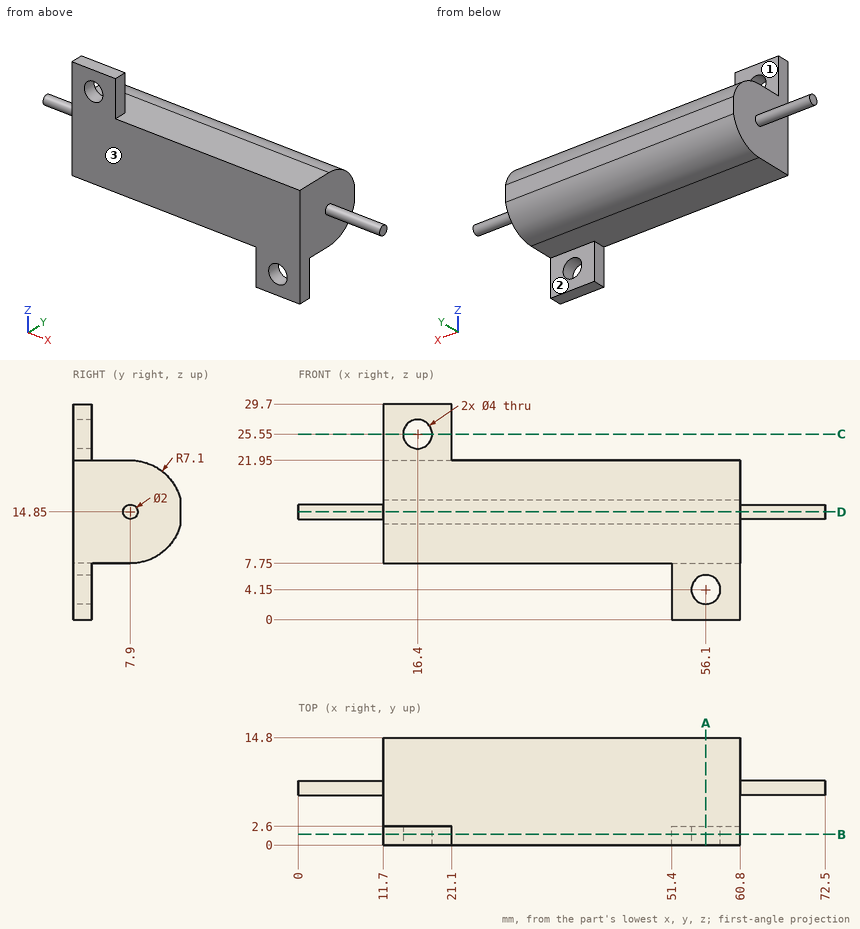
Design review of the part shown in the three views and the two pictorial views. Dimensions are in mm from the part's minimum x, y and z. A direction names the side the tool comes from. Coordinates: 2 decimals unless noted, no trailing zeros. Write each loop counter-clockwise with the first axis right and the second up, starting at its lowest first coordinate (ties: lowest second). Pieces come first, ordered by that corner, then holes. Notation, with made-up numbers: (-20, 84) - (35, 84) arc R13 ccw to (35, 99) - close; hole circle Ø5 at (-19.75, -7). An arc over 180 degrees is marked (long way). Write item = value, one per line.
(1) For P1, Ø4.5, axis at y = 5.5, z = 23, coming from the -X side; P2, Ø1.3, axis at y = 2, z = 24.5, coming from the +X side; P3, Ø3, axis at x = 54.5, y = 6, coming from the -Z side; P4, Ø3, axis at x = 56.1, z = 4.15, coming from the +Y side, all flat-tipped, find the tip position at first contact; note any pin that passes through.
Result sheet:
P1 = 11.7
P2 = 21.1
P3 = 7.75
P4 = through
(2) Consider section B-B, the plane y = 1.5. Give the boundary of the cut face in (x, z), then the cut area to 3 significant figures.
Result sheet:
outline = (11.7, 7.75) - (51.4, 7.75) - (51.4, 0) - (60.8, 0) - (60.8, 21.95) - (21.1, 21.95) - (21.1, 29.7) - (11.7, 29.7) - close; hole circle Ø4 at (16.4, 25.55); hole circle Ø4 at (56.1, 4.15)
area = 818 mm^2
(3) For line 1 (Z direction, x = 16.4, y = 1); line 2 (Z direction, x = 38, y = 1.5); line 3 (X direction, y = 3.25, z = 18.5), list the stretches that pass through material, from the lowest coordinate up. Write a range as [from, to].
Result sheet:
line_1 = [7.75, 23.55], [27.55, 29.7]
line_2 = [7.75, 21.95]
line_3 = [11.7, 60.8]
(4) Consider section D-D, the plane z = 14.85. Give the boundary of the cut face in (x, y).
Result sheet:
outline = (0, 6.9) - (11.7, 6.9) - (11.7, 0) - (60.8, 0) - (60.8, 6.9) - (72.5, 6.9) - (72.5, 8.9) - (60.8, 8.9) - (60.8, 14.8) - (11.7, 14.8) - (11.7, 8.9) - (0, 8.9) - close
(5) Consider section A-A, the plane x = 56.1. Give the boundary of the cut face in (y, z).
Result sheet:
outline = (0, 0) - (2.6, 0) - (2.6, 2.15) - (0, 2.15) - close; (0, 6.15) - (2.6, 6.15) - (2.6, 7.75) - (7.9, 7.75) arc R7.1 ccw to (14.8, 13.18) - (14.8, 16.52) arc R7.1 ccw to (7.9, 21.95) - (0, 21.95) - close
(6) Machinability: for the marked faces 1, 2 and 3, which of the approach directions +Z, -Z, +X, -X, +Y, -Y give a long, thin tool a straight path to every point of the face, cutting with its end or side? Answer none if there is none.
Result sheet:
face_1 = +Z, +X, -X, +Y
face_2 = -Z, +X, -X, +Y
face_3 = +Z, -Z, +X, -X, -Y
(7) Consider section C-C, the plane z = 25.55. Give the boundary of the cut face in (x, y), then the cut area to 3 significant figures.
Result sheet:
outline = (11.7, 0) - (14.4, 0) - (14.4, 2.6) - (11.7, 2.6) - close; (18.4, 0) - (21.1, 0) - (21.1, 2.6) - (18.4, 2.6) - close
area = 14.0 mm^2
